```python
from build123d import *

# Parameters (mm, degrees)
SKETCH2_R           = 110
BOSS_EXTRUDE2_DEPTH = 10
SKETCH4_R           = 9.5
CUT_EXTRUDE1_DEPTH  = 6
SKETCH6_R           = 4
CUT_EXTRUDE3_DEPTH  = 156.679157243
SKETCH7_R           = 2
CUT_EXTRUDE6_DEPTH  = 156.884572681
SKETCH8_R           = 2
CUT_EXTRUDE7_DEPTH  = 10


with BuildPart() as part:
    # Sketch2 → Boss-Extrude2 (new body)
    with BuildSketch(Plane(origin=(0, 0, 0), x_dir=(1, 0, 0), z_dir=(0, 1, 0))):
        with Locations(Location((0, 0, 0), (0, 0, 270))):
            Circle(SKETCH2_R)
    extrude(amount=BOSS_EXTRUDE2_DEPTH)

    # Sketch4 → Cut-Extrude1 (cut)
    with BuildSketch(Plane(origin=(0, 0, 0), x_dir=(-1, 0, 0), z_dir=(0, -1, 0))):
        with Locations(Location((0, 0, 0), (0, 0, 90))):
            Circle(SKETCH4_R)
    extrude(amount=-CUT_EXTRUDE1_DEPTH, mode=Mode.SUBTRACT)

    # Sketch6 → Cut-Extrude3 (cut, through all)
    with BuildSketch(Plane(origin=(0, 6, 0), x_dir=(-1, 0, 0), z_dir=(0, -1, 0))):
        with Locations(Location((0, 0, 0), (0, 0, 90))):
            Circle(SKETCH6_R)
    extrude(amount=-CUT_EXTRUDE3_DEPTH, mode=Mode.SUBTRACT)

    # Sketch7 → Cut-Extrude6 (cut, through all)
    with BuildSketch(Plane(origin=(0, 0, 0), x_dir=(-1, 0, 0), z_dir=(0, -1, 0))):
        with Locations(Location((32, -17.5, 0), (0, 0, 90))):
            Circle(SKETCH7_R)
        with Locations(Location((32, 17.5, 0), (0, 0, 90))):
            Circle(SKETCH7_R)
        with Locations(Location((-32, 17.5, 0), (0, 0, 90))):
            Circle(SKETCH7_R)
        with Locations(Location((-32, -17.5, 0), (0, 0, 90))):
            Circle(SKETCH7_R)
    extrude(amount=-CUT_EXTRUDE6_DEPTH, mode=Mode.SUBTRACT)

    # Sketch8 → Cut-Extrude7 (cut)
    with BuildSketch(Plane.XZ):
        with Locations(Location((0, 95, 0), (0, 0, 270))):
            Circle(SKETCH8_R)
        with Locations(Location((67.175144213, 67.175144213, 0), (0, 0, 270))):
            Circle(SKETCH8_R)
        with Locations(Location((95, 0, 0), (0, 0, 270))):
            Circle(SKETCH8_R)
        with Locations(Location((67.175144213, -67.175144213, 0), (0, 0, 270))):
            Circle(SKETCH8_R)
        with Locations(Location((0, -95, 0), (0, 0, 270))):
            Circle(SKETCH8_R)
        with Locations(Location((-67.175144213, -67.175144213, 0), (0, 0, 270))):
            Circle(SKETCH8_R)
        with Locations(Location((-95, 0, 0), (0, 0, 270))):
            Circle(SKETCH8_R)
        with Locations(Location((-67.175144213, 67.175144213, 0), (0, 0, 270))):
            Circle(SKETCH8_R)
    extrude(amount=-CUT_EXTRUDE7_DEPTH, mode=Mode.SUBTRACT)


solid = part.part
```
The model under review builds one solid part; all positions refer to its coordinate system, in mm. A direction names the side the tool comes from. Coordinates: 2 decimals unless noted, no trailing zeros. Loops run counter-clockwise (first coordinate to the right, second up) from the corner with the lowest first, then second, coordinate; pieces in that order, holes last. Notation, with made-up numbers: (34.25, 10) -> (78.25, 10) arc R8 cw to (78.25, 20) -> close; hole circle Ø1 at (-3, 10). An arc over 180 degrees is marked (long way). Answer as CSV lines item,"result".
Item 1: Insertion check: pin 1 (1 mm diameter, centred on x = -9, y = 3.5, fed in from -Z); pin 2 (2 mm diameter, centred on x = -36, y = 8, fed in from -Z); pin 3 (5 mm diameter, centred on y = 5.5, z = -41.5, fed in from -X). Each pin has a flat end and moves straight along its axis. Give the tip position at first contact, or say it passes through.
Results below:
pin 1,"stops at z = -109.67"
pin 2,"stops at z = -104.28"
pin 3,"stops at x = -102.85"
Item 2: Draft analysis for pull direction X (two halves, no side actions). For faces 1 (the cylindrical face through (-97.59, 4.93, 50.76)), 2 (the cylindrical face through (-5.78, 2.96, 7.54)), 3 (the cylindrical face through (-3.905, 7.972, 0.867)), 4 (the flat face through (-23, 0, -2)), state which applies: +X half, -X half, draft (parallel to the pull), parting line (faces both ways), or undercut.
Results below:
face 1,"parting line"
face 2,"undercut"
face 3,"undercut"
face 4,"draft"
Item 3: Take a section at A-A, the plane z = -60. State the section outline as (x, y) points.
Results below:
outline,"(-92.2, 0) -> (92.2, 0) -> (92.2, 10) -> (-92.2, 10) -> close"
Item 4: Machinability: for faces 5 (the flat face through (-23, 10, -2)), 6 (the flat face through (-4, 6, -2)), which of the approach directions +Z, -Z, +X, -X, +Y, -Y give a long, thin tool a straight path to every point of the face, cutting with its end or side? Answer none if there is none.
Results below:
face 5,"+Z, -Z, +X, -X, +Y"
face 6,"-Y"
Item 5: Take a section at B-B, the plane x = 22.5. State the section outline as (y, z) points, and give its area (3 significant figures).
Results below:
outline,"(0, -107.67) -> (10, -107.67) -> (10, 107.67) -> (0, 107.67) -> close"
area,"2,150 mm2"
Item 6: For L1, parallel to X at y = 4.15, z = 0; L2, parallel to Z at x = 68, y = 5.75; L3, parallel to Z at x = 68.5, y = 2, list the stretches that pass through material, from the lowest coordinate up.
Results below:
L1,"x = -110 to -97, -93 to -9.5, 9.5 to 93, 97 to 110"
L2,"z = -86.46 to -69, -65.35 to 65.35, 69 to 86.46"
L3,"z = -86.07 to -68.67, -65.68 to 65.68, 68.67 to 86.07"
